Verification items for the finished model (mm, model axes). Face numbers are marked on the shaded views. A direction names the side the tool comes from. Coordinates: 2 decimals unless noted, no trailing zeros. Write each loop counter-clockwise with the first axis right and the second up, starting at its lowest first coordinate (ties: lowest second). Pieces come first, ordered by that corner, then holes. Notation, with made-up numbers: (52.5, -26.75) -> (98.5, -26.75) arc R32 cw to (98.5, 11.25) -> close; hole circle Ø5 at (32.5, 77). An arc over 180 degrees is marked (long way). Use a Markdown table: item, result. Add a question column.
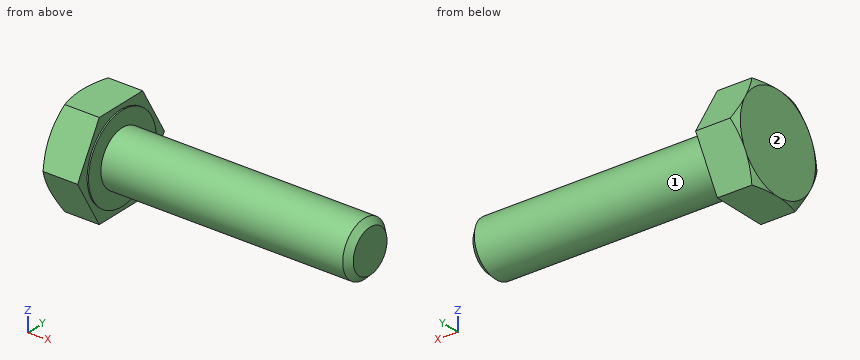
Autodesk Inventor part; units mm, degrees
ref_plane "Work Plane1" through (1.525, 0, 0) normal (0, 0, 1) x (1, 0, 0)
ref_plane "YZ Plane" through (0, 0, 0) normal (1, 0, 0) x (0, 1, 0)
ref_plane "XZ Plane" through (0, 0, 0) normal (0, 1, 0) x (-1, 0, 0)
sketch "Szkic1" plane through (0, 0, 0) normal (0, 0, 1) x (1, 0, 0)
  line L0 (0, 3.15) -> (0, 2)
  line L1 (4, 2) -> (18, 2)
  line L2 (18, 2) -> (18, 0)
  line L3 (18, 0) -> (-0.1001, 0)
  line L4 (-3.7201, 0) -> (21.62, 0)
  line L5 (-0.1001, 0) -> (-0.1001, 3.15)
  line L6 (-0.1001, 3.15) -> (0, 3.15)
  line L7 (4, 2) -> (3.5705, 2)
  line L8 (3.5705, 2) -> (0, 2)
  line L9 (0, -0.63) -> (0, 3.78)
  dimension "d0" = 18
  dimension "d1" = 14
  dimension "d2" = 4
  dimension "d9" = 0.1001
  dimension "d10" = 6.3
  dimension "d13" = 0.4295
  dimension "d14" = 4
revolve "Bryła" add sketch "Szkic1" angle 360 about axis through (18, 0, 0) along (-1, 0, 0)
sketch "Szkic2" plane through (-0.1001, 0, 0) normal (-1, 0, 0) x (0, 0, 1)
  line L0 (0, 4.0415) -> (3.5, 2.0207)
  line L1 (3.5, 2.0207) -> (3.5, -2.0207)
  line L2 (3.5, -2.0207) -> (0, -4.0415)
  line L3 (0, -4.0415) -> (-3.5, -2.0207)
  line L4 (-3.5, -2.0207) -> (-3.5, 2.0207)
  line L5 (-3.5, 2.0207) -> (0, 4.0415)
  point P0 (0, 0)
  point P1 (0, 0)
  dimension "d11" = 7
extrude "Głowica" add sketch "Szkic2" along normal blind 2.825
sketch "Szkic4" plane through (0, 0, 0) normal (0, 0, 1) x (1, 0, 0)
  line L0 (-2.9251, 3.5) -> (-2.9251, 4.0415)
  line L1 (-2.9251, 4.0415) -> (-2.6125, 4.0415)
  line L2 (-2.6125, 4.0415) -> (-2.9251, 3.5)
  line L3 (-3.4901, 0) -> (0.4649, 0)
  line L4 (-0.1001, 4.0415) -> (-2.9251, 4.0415)
  line L5 (-2.9251, 2.0207) -> (-2.9251, 4.0415)
  dimension "d5" = 30
  dimension "d19" = 7
revolve "Faza1" cut sketch "Szkic4" angle 360 about axis through (-10, 0, 0) along (1, 0, 0)
thread "Gwint"
chamfer "Faza2" distance 0.4294 distance2 0.4295 1 edges at (18, -2, 0) measured on face at (18, -0.499, 0.4421)
ref_plane "Work Plane1" through (1.525, 0, 0) normal (0, 0, 1) x (1, 0, 0)
equation "\"d0\" = NLG"
equation "\"d1\" = GEL"
equation "\"d2\" = GD"
equation "\"d10\" = SD2"
equation "\"d14\" = BDM"
equation "\"d11\" = SW"
equation "\"d3\" = KOH - SD"
equation "\"d5\" = ANG1"
equation "\"d19\" = SW0"
equation "\"d15\" = GEL"
equation "\"d6\" = -0.5 * SPD + 0.5 * GD"
equation "\"NLG\" = 18"
equation "\"GD\" = NND"
equation "\"BDM\" = NND"
equation "\"KOH\" = 2.925"
equation "\"GEL\" = 14"
equation "\"SW\" = 7"
equation "\"SW0\" = 7"
equation "\"SPD\" = NND - 1.2269 * PTC"
equation "\"SD2\" = 0.9 * SW"
equation "\"SD\" = 0.1"
equation "\"ANG1\" = 30deg"
equation "\"GAL\" = 0.61345 * PTC"
equation "\"GUL\" = 0.61345 * PTC"
equation "\"RR\" = 0.35"
equation "\"GD1\" = THREADDIA - 1.2269 * PTC"
equation "\"THREADDIA\" = 4"
equation "\"SDH\" = 6.55"
equation "\"TOA\" = 30deg"
equation "\"PTC\" = 0.7"
equation "\"NND\" = 4"
equation "\"E0\" = 1.155 * SW"
properties part number "BS 3692 - M4 x 18" material "Stal, miękka"
1) Set-up check for the marked faces 1 and 2: record each of +Z, -Z, +X, -X, +Y, -Y from which the full face is reachable in a straight line by a thin tool's end or side.
2) Thickness scan on L1, parallel to X at y = -2.25, z = -1.75; L2, parallel to Y at x = -0.75, z = -1.5; L3, parallel to Y at x = 10, z = -0.5. Record the ranges inside material, lowest first.
3) Cross-section at A-A on x = 13.75. Record the boundary of the cut face in (y, z).
4) Gauge pin test, flat end, axial feed: pin 1 (2 mm diameter, centred on x = 11, z = 0, fed in from -Y). Record the tip position at first contact, or that the pin passes through.
Returned:
| question | item | result |
|---|---|---|
| 1 | face 1 | +X |
| 1 | face 2 | +Z, -Z, -X, +Y, -Y |
| 2 | L1 | x = -2.93 to 0 |
| 2 | L2 | y = -3.18 to 3.18 |
| 2 | L3 | y = -1.94 to 1.94 |
| 3 | outline | circle Ø4 at (0, 0) |
| 4 | pin 1 | stops at y = -2 |
